Read the model definition and answer for the solid it produces. Units are mm, in the model's axes. Give positions to 0.01 mm unless a question says otherwise; leave off trailing zeros. Write each loop counter-clockwise with the first axis right and the second up, starting at its lowest first coordinate (ties: lowest second). Pieces come first, ordered by that corner, then holes. Notation, with made-up numbers: (66.5, 15) -> (81.5, 15) arc R25 ccw to (81.5, 46) -> close; hole circle Ø6 at (6, 1). An arc over 180 degrees is marked (long way). Use a Markdown table: item, result.
from build123d import *

# Parameters (mm, degrees)
SKETCH1_R             = 5
BODY_DEPTH            = 9
PIN_INSERT_DEPTH      = 12.445523142
PIN_INSERT_DEPTH_BACK = 12.445523142
SKETCH2_R             = 1.5
HEAD_SA_R             = 1.784


with BuildPart() as part:
    # Sketch1 → body (new body)
    with BuildSketch(Plane(origin=(0, 0, 0), x_dir=(1, 0, 0), z_dir=(0, 1, 0))):
        with Locations(Location((0, 0, 0), (0, 0, 270))):
            Circle(SKETCH1_R)
    extrude(amount=BODY_DEPTH)

    # Sketch2 → pin insert (cut, two sides: drawn at the far end of the back side and taken through both)
    with BuildSketch(Plane(origin=(0, 0, 0), x_dir=(0, 0, -1), z_dir=(1, 0, 0)).offset(-PIN_INSERT_DEPTH_BACK)):
        with Locations((0, 2)):
            Circle(SKETCH2_R)
    extrude(amount=PIN_INSERT_DEPTH + PIN_INSERT_DEPTH_BACK, mode=Mode.SUBTRACT)

    # head SA → section 0 of cone
    with BuildSketch(Plane(origin=(0, 19, 0), x_dir=(1, 0, 0), z_dir=(0, 1, 0)), mode=Mode.PRIVATE) as cone_s0:
        Circle(HEAD_SA_R)
    # loft up to a face of the part (cone)
    loft([cone_s0.sketch, part.faces().sort_by_distance((0, 9, 0))[0]])


solid = part.part
Item 1: A cutting plane is placed at C-C (y = 2). Give the vertices of the cut face in (x, z), then the cut area to 3 significant figures.
Return value:
| item | result |
|---|---|
| outline | (-4.77, -1.5) arc R5 ccw to (4.77, -1.5) -> close; (-4.77, 1.5) -> (4.77, 1.5) arc R5 ccw to start |
| area | 49.0 mm^2 |
Item 2: Straight lines are drawn through the part: line 1 along Y through (x, z) = (0.5, 0); line 2 along Z through (x, y) = (-1.75, 2); line 3 along Z through (x, y) = (-3, 2.75). For each, find the intervals that lie inside material, in ascending order. Write a range as [from, to].
Return value:
| item | result |
|---|---|
| line 1 | [0, 0.5], [3.5, 19] |
| line 2 | [-4.68, -1.5], [1.5, 4.68] |
| line 3 | [-4, -1.3], [1.3, 4] |
Item 3: For a pull along Y with two mould halves and no side action, classify faces 1 (the face through (0, 19, 0)), 2 (the face through (-0.07, 0.536, 0.325)), 3 (the face through (0, 0, 0)) as +Y half, -Y half, draft (parallel to the pull), parting line (faces both ways), or undercut.
Return value:
| item | result |
|---|---|
| face 1 | +Y half |
| face 2 | undercut |
| face 3 | -Y half |
Item 4: A cutting plane is placed at A-A (x = 0). Give the vertices of the cut face in (y, z).
Return value:
| item | result |
|---|---|
| outline | (0, -5) -> (9, -5) -> (19, -1.78) -> (19, 1.78) -> (9, 5) -> (0, 5) -> close; hole circle Ø3 at (2, 0) |
Item 5: A cutting plane is placed at B-B (y = 7.25). Give the vertices of the cut face in (x, z), then the cut area to 3 significant figures.
Return value:
| item | result |
|---|---|
| outline | circle Ø10 at (0, 0) |
| area | 78.5 mm^2 |
Item 6: Each of these flat-tipped pins is pushed along its axis until it touches: P1, Ø1.5, axis at y = 10.5, z = 0, coming from the -X side; P2, Ø2, axis at y = 12.5, z = 2.5, coming from the +X side. Where does it stop, or does it pass through?
Return value:
| item | result |
|---|---|
| P1 | x = -4.76 |
| P2 | x = 3.7 |
Item 7: A cutting plane is placed at D-D (y = 17.5). Give the vertices of the cut face in (x, z), then the cut area to 3 significant figures.
Return value:
| item | result |
|---|---|
| outline | circle Ø4.53 at (0, 0) |
| area | 16.1 mm^2 |
